```python
from build123d import *

# Parameters (mm, degrees)
SKETCH1_W           = 30
SKETCH1_H           = 55
BOSS_EXTRUDE1_DEPTH = 10
CUT_EXTRUDE1_DEPTH  = 58.879184514
CUT_EXTRUDE3_DEPTH  = 42.907636536
SKETCH9_W           = 5
SKETCH9_H           = 30
CUT_EXTRUDE4_DEPTH  = 10


with BuildPart() as part:
    # Sketch1 → Boss-Extrude1 (new body)
    with BuildSketch(Plane(origin=(0, 0, 0), x_dir=(1, 0, 0), z_dir=(0, 1, 0))):
        Rectangle(SKETCH1_W, SKETCH1_H)
    extrude(amount=BOSS_EXTRUDE1_DEPTH)

    # Sketch6 → Cut-Extrude1 (cut, through all)
    with BuildSketch(Plane(origin=(0, 0, -27.5), x_dir=(-1, 0, 0), z_dir=(0, 0, -1))):
        with BuildLine():
            Line((-8, 7.3), (-9.647377045, 6.605038589))
            ThreePointArc((-9.647377045, 6.605038589), (-8, 2.7), (-6.352622955, 6.605038589))
            Line((-6.352622955, 6.605038589), (-8, 7.3))
        make_face()
        with BuildLine():
            Line((8, 7.3), (6.243284106, 6.484570399))
            ThreePointArc((6.243284106, 6.484570399), (8, 2.7), (9.756715894, 6.484570399))
            Line((9.756715894, 6.484570399), (8, 7.3))
        make_face()
    extrude(amount=-CUT_EXTRUDE1_DEPTH, mode=Mode.SUBTRACT)

    # Sketch8 → Cut-Extrude3 (cut, through all)
    with BuildSketch(Plane(origin=(15, 0, 0), x_dir=(0, 0, -1), z_dir=(1, 0, 0))):
        with BuildLine():
            Line((10.5, 7.3), (12.417920009, 6.269481327))
            ThreePointArc((12.417920009, 6.269481327), (10.5, 2.7), (8.582079991, 6.269481327))
            Line((8.582079991, 6.269481327), (10.5, 7.3))
        make_face()
    extrude(amount=-CUT_EXTRUDE3_DEPTH, mode=Mode.SUBTRACT)

    # Sketch9 → Cut-Extrude4 (cut)
    with BuildSketch(Plane.XZ):
        with Locations((0, -12.5)):
            Rectangle(SKETCH9_W, SKETCH9_H)
    extrude(amount=-CUT_EXTRUDE4_DEPTH, mode=Mode.SUBTRACT)


solid = part.part
```
Input: part model. Units: mm. Frame: model coordinates. A direction names the side the tool comes from. Give positions to 0.01 mm unless a question says otherwise; leave off trailing zeros. Order: outer loops, then holes, each group sorted by start corner. A loop starts at its lowest first (then second) coordinate and runs counter-clockwise, first axis right, second up. Notation, with made-up numbers: (58.25, 37) - (110.25, 37) arc R22 ccw to (110.25, 45) - close; hole circle Ø6 at (30, -27). An arc over 180 degrees is marked (long way). Use a Markdown table: item, result.
(1) Line query: line 1 (X direction, y = 5, z = -19.75); line 2 (X direction, y = 2.5, z = -14); line 3 (Z direction, x = -12.25, y = 5). Output: solid intervals per line, ascending. Write a range as from..to.
Computed values:
| item | result |
|---|---|
| line 1 | x = -15..-10.3, -5.7..-2.5, 2.5..5.7, 10.3..15 |
| line 2 | x = -15..-2.5, 2.5..15 |
| line 3 | z = -27.5..-12.8, -8.2..27.5 |
(2) Draft query along Y for faces 4 (the flat face through (-2.5, 4, -13)), 5 (the cylindrical face through (12.33, 2.7, -10.57)), 6 (the flat face through (-4, 10, 0)), 7 (the flat face through (-7.134, 6.898, 8.234)). Return one class per face: released by +Y, released by -Y, zero draft, split by the parting line, or undercut.
Computed values:
| item | result |
|---|---|
| face 4 | zero draft |
| face 5 | undercut |
| face 6 | released by +Y |
| face 7 | undercut |
(3) Pin query (flat end, axial travel): pin 1 (4 mm diameter, centred on x = 0, y = 5.5, fed in from -Z). Return the tip coordinate at first contact, or that it passes through.
Computed values:
| item | result |
|---|---|
| pin 1 | stops at z = 2.5 |
(4) Section query B-B (y = 5). State how many separate pieces and enclosed holes the cut face has, then the cut area to 3 significant figures.
Computed values:
| item | result |
|---|---|
| separate pieces | 7 |
| enclosed holes | 0 |
| area | 921 mm2 |
(5) Section query C-C (x = 11). Output: boundary loops of the cut face in (y, z).
Computed values:
| item | result |
|---|---|
| outline | (0, -27.5) - (10, -27.5) - (10, 27.5) - (0, 27.5) - close; hole (6.27, -12.42) - (7.3, -10.5) - (6.27, -8.58) arc R2.3 ccw (long way) to start |
(6) Section query A-A (z = -18). Output: boundary loops of the cut face in (x, y), then the cut area to 3 significant figures.
Computed values:
| item | result |
|---|---|
| outline | (-15, 0) - (-2.5, 0) - (-2.5, 10) - (-15, 10) - close; (2.5, 0) - (15, 0) - (15, 10) - (2.5, 10) - close; hole (-9.76, 6.48) arc R2.3 ccw (long way) to (-6.24, 6.48) - (-8, 7.3) - close; hole (6.35, 6.61) arc R2.3 ccw (long way) to (9.65, 6.61) - (8, 7.3) - close |
| area | 218 mm2 |
(7) Access query for faces 1 (the flat face through (8.81, 6.96, -19.12)), 2 (the flat face through (-10.2, 3.8, -27.5)), 3 (the flat face through (-12.23, 6.79, -11.45)). Directions: +Z, -Z, +X, -X, +Y, -Y. A direction counts if a zero-diameter tool reaches every point of the face in a straight line with its end or side. Return the directions, or none.
Computed values:
| item | result |
|---|---|
| face 1 | +Z, -Z |
| face 2 | -Z, +X, -X, +Y, -Y |
| face 3 | +X, -X |
(8) Section query D-D (z = 12). Output: boundary loops of the cut face in (x, y).
Computed values:
| item | result |
|---|---|
| outline | (-15, 0) - (15, 0) - (15, 10) - (-15, 10) - close; hole (-9.76, 6.48) arc R2.3 ccw (long way) to (-6.24, 6.48) - (-8, 7.3) - close; hole (6.35, 6.61) arc R2.3 ccw (long way) to (9.65, 6.61) - (8, 7.3) - close |
